from build123d import *

# Parameters (mm, degrees)
SKETCH1_R           = 26
BOSS_EXTRUDE1_DEPTH = 4
SKETCH2_R           = 3.1
CUT_EXTRUDE1_DEPTH  = 4
SKETCH4_R           = 16
SKETCH4_R_2         = 13
BOSS_EXTRUDE2_DEPTH = 2.5
CHAMFER1_SIZE       = 0.5
CHAMFER2_SIZE       = 0.5


with BuildPart() as part:
    # Sketch1 → Boss-Extrude1 (new body)
    with BuildSketch(Plane.XY):
        Circle(SKETCH1_R)
    extrude(amount=BOSS_EXTRUDE1_DEPTH)

    # Sketch2 → Cut-Extrude1 (cut)
    with BuildSketch(Plane.XY.offset(4)):
        with Locations((21, 0)):
            Circle(SKETCH2_R)
        with Locations((-10.5, -18.186533479)):
            Circle(SKETCH2_R)
        with Locations((-10.5, 18.186533479)):
            Circle(SKETCH2_R)
    extrude(amount=-CUT_EXTRUDE1_DEPTH, mode=Mode.SUBTRACT)

    # Sketch4 → Boss-Extrude2 (add)
    with BuildSketch(Plane.XY.offset(4)):
        Circle(SKETCH4_R)
        Circle(SKETCH4_R_2, mode=Mode.SUBTRACT)
    extrude(amount=BOSS_EXTRUDE2_DEPTH)

    # Chamfer1
    chamfer1_edges = [part.edges().sort_by_distance(p)[0] for p in [
        (-16, 0, 6.5),
    ]]
    chamfer(chamfer1_edges, length=CHAMFER1_SIZE)

    # Chamfer2
    chamfer2_edges = [part.edges().sort_by_distance(p)[0] for p in [
        (-13, 0, 6.5),
    ]]
    chamfer(chamfer2_edges, length=CHAMFER2_SIZE)


solid = part.part
The listing builds one solid part. Answer for the finished solid, in the listing's coordinates (mm). A direction names the side the tool comes from. Round coordinates to 2 decimals unless told otherwise and drop trailing zeros. Write each loop counter-clockwise with the first axis right and the second up, starting at its lowest first coordinate (ties: lowest second). Pieces come first, ordered by that corner, then holes. Notation, with made-up numbers: (31, 78.25) - (65, 78.25) arc R26 cw to (65, 93.25) - close; hole circle Ø3 at (33.5, 27). An arc over 180 degrees is marked (long way). Use a Markdown table: item, result. Add a question column.
1. Flat-ended cylindrical pins translate along their axes: P1, Ø3, axis at y = 9, z = 2, coming from the +X side; P2, Ø1.5, axis at y = 12, z = 2.5, coming from the +X side; P3, Ø1.5, axis at x = 18.5, y = 8, coming from the -Z side; P4, Ø1.5, axis at y = -3, z = 0.5, coming from the -X side. Find the tip coordinate at first contact, or state that the pin passes through.
2. The part is cut by section A-A (y = 0). Write down the section's boundary in (x, z).
3. A tool of negligible diameter and unlimited length cuts with its end or side. For faces 1 (the face through (-5, 13, 6.5)), 2 (the face through (-3.47, -15.62, 4.99)), from which of +Z, -Z, +X, -X, +Y, -Y can it reach the whole face along a straight path? Write none if from no direction.
4. The part is cut by section B-B (x = 21). Write down the section's boundary in (y, z).
5. For a pull along Y with two mould halves and no side action, classify faces 3 (the face through (0, 0, 0)), 4 (the face through (-20.633, -15.821, 1.972)), 5 (the face through (-10.316, -7.91, 4.986)) as +Y half, -Y half, draft (parallel to the pull), parting line (faces both ways), or undercut.
6. The part is cut by section C-C (x = 0). Write down the section's boundary in (y, z), and give its area (4 significant figures).
7. The part is cut by section D-D (z = 5.25). Write down the section's boundary in (x, y).
8. Consider line 1 (Y direction, x = 0, z = 4.5); line 2 (Y direction, x = -10.5, z = 2.65); line 3 (X direction, y = -20, z = 3). Determine where each line is inside the solid, lowest interval first.
Reported:
| question | item | result |
|---|---|---|
| 1 | P1 | x = 24.89 |
| 1 | P2 | x = 23.44 |
| 1 | P3 | z = 0 |
| 1 | P4 | x = -25.9 |
| 2 | outline | (-26, 0) - (17.9, 0) - (17.9, 4) - (16, 4) - (16, 6) - (15.5, 6.5) - (13.5, 6.5) - (13, 6) - (13, 4) - (-13, 4) - (-13, 6) - (-13.5, 6.5) - (-15.5, 6.5) - (-16, 6) - (-16, 4) - (-26, 4) - close; (24.1, 0) - (26, 0) - (26, 4) - (24.1, 4) - close |
| 3 | face 1 | +Z, +X, -X, +Y, -Y |
| 3 | face 2 | +Z |
| 4 | outline | (-15.33, 0) - (-3.1, 0) - (-3.1, 4) - (-15.33, 4) - close; (3.1, 0) - (15.33, 0) - (15.33, 4) - (3.1, 4) - close |
| 5 | face 3 | draft |
| 5 | face 4 | parting line |
| 5 | face 5 | undercut |
| 6 | outline | (-26, 0) - (26, 0) - (26, 4) - (16, 4) - (16, 6) - (15.5, 6.5) - (13.5, 6.5) - (13, 6) - (13, 4) - (-13, 4) - (-13, 6) - (-13.5, 6.5) - (-15.5, 6.5) - (-16, 6) - (-16, 4) - (-26, 4) - close |
| 6 | area | 222.5 mm^2 |
| 7 | outline | circle Ø32 at (0, 0); hole circle Ø26 at (0, 0) |
| 8 | line 1 | -16 to -13, 13 to 16 |
| 8 | line 2 | -23.79 to -21.29, -15.09 to 15.09, 21.29 to 23.79 |
| 8 | line 3 | -16.61 to -13.01, -7.99 to 16.61 |
